from build123d import *

# Parameters (mm, degrees)
F1_DEPTH     = 155
F2_R         = 5
F3_T1_DEPTH  = 145
F3_T3_DEPTH  = 28.172866076
F3_T5_DEPTH  = 18.1728662684
F3_T8_ANGLE  = 90
F3_T10_ANGLE = 90
F3_T12_ANGLE = 88.5674563985
F3_T14_ANGLE = 88.5674563985
F4_R         = 2
F5_R         = 1
F6_R         = 1


# Not quite as in the source:
# - a fillet or chamfer that OpenCascade refuses, or shapes differently, is made with other operations: its cross-section is extruded or revolved along the edge and cut away or added


with BuildPart() as f1:
    # F0 (on Top) → F1 (new body)
    with BuildSketch(Plane.XY):
        Polygon((-2.000000095, 0), (0, 0), (0, 30), (18, 30), (18.999999905, 69.9874980486), (17.0006250026, 70.0374980439), (16.0493903369, 32.000000095), (-2.000000095, 32.000000095), align=None)
    extrude(amount=F1_DEPTH)

    # F2
    f2_edges = [f1.edges().sort_by_distance(p)[0] for p in [
        (16.04939, 32, 77.5),
        (18.000312, 70.012498, 155),
        (18.000312, 70.012498, 0),
    ]]
    fillet(f2_edges, radius=F2_R)

    # F3: fillet of radius 2 on 6 edges, made by hand

    # F3_s2 → F3_t1 (cut)
    with BuildSketch(Plane.XY.offset(5)):
        with BuildLine():
            ThreePointArc((18.999999905, 69.9874980486), (17.5715836938, 69.4372500336), (16.9506250073, 68.0381231415))
            Line((16.9506250073, 68.0381231415), (17.0006250026, 70.0374980439))
            Line((17.0006250026, 70.0374980439), (18.999999905, 69.9874980486))
        make_face()
    extrude(amount=F3_T1_DEPTH, mode=Mode.SUBTRACT)

    # F3_s4 → F3_t3 (cut)
    with BuildSketch(Plane(origin=(1.6360154319, 65.4201701064, 0), x_dir=(0, 0, 1), z_dir=(-0.0249999976, -0.9996874512, 0))):
        with BuildLine():
            ThreePointArc((0, -17.2443741931), (0.5857864376, -15.8301606308), (2, -15.2443741931))
            Line((2, -15.2443741931), (0, -15.2443741931))
            Line((0, -15.2443741931), (0, -17.2443741931))
        make_face()
        with BuildLine():
            ThreePointArc((155, -17.2443741931), (154.4142135624, -15.8301606308), (153, -15.2443741931))
            Line((153, -15.2443741931), (155, -15.2443741931))
            Line((155, -15.2443741931), (155, -17.2443741931))
        make_face()
    extrude(amount=F3_T3_DEPTH, mode=Mode.SUBTRACT)

    # F3_s6 → F3_t5 (cut)
    with BuildSketch(Plane.YZ.offset(-7.000000095)):
        with BuildLine():
            ThreePointArc((30.000000095, 155), (31.4142136574, 154.4142135624), (32.000000095, 153))
            Line((32.000000095, 153), (32.000000095, 155))
            Line((32.000000095, 155), (30.000000095, 155))
        make_face()
        with BuildLine():
            ThreePointArc((30.000000095, 0), (31.4142136574, 0.5857864376), (32.000000095, 2))
            Line((32.000000095, 2), (32.000000095, 0))
            Line((32.000000095, 0), (30.000000095, 0))
        make_face()
    extrude(amount=F3_T5_DEPTH, mode=Mode.SUBTRACT)

    # F3_s7 → F3_t8 (revolve, cut)
    with BuildSketch(Plane.XY.offset(5)):
        with BuildLine():
            ThreePointArc((18.999999905, 69.9874980486), (17.5715836938, 69.4372500336), (16.9506250073, 68.0381231415))
            Line((16.9506250073, 68.0381231415), (17.0006250026, 70.0374980439))
            Line((17.0006250026, 70.0374980439), (18.999999905, 69.9874980486))
        make_face()
    revolve(axis=Axis((16.8756250144, 65.0390607878, 5), (-0.9996874512, 0.0249999976, 0)), revolution_arc=F3_T8_ANGLE, mode=Mode.SUBTRACT)

    # F3_s9 → F3_t10 (revolve, cut)
    with BuildSketch(Plane.XY.offset(150)):
        with BuildLine():
            ThreePointArc((18.999999905, 69.9874980486), (17.5715836938, 69.4372500336), (16.9506250073, 68.0381231415))
            Line((16.9506250073, 68.0381231415), (17.0006250026, 70.0374980439))
            Line((17.0006250026, 70.0374980439), (18.999999905, 69.9874980486))
        make_face()
    revolve(axis=Axis((16.8756250144, 65.0390607878, 150), (0.9996874512, -0.0249999976, 0)), revolution_arc=F3_T10_ANGLE, mode=Mode.SUBTRACT)

    # F3_s11 → F3_t12 (revolve, cut)
    with BuildSketch(Plane(origin=(0.9316938469, 37.2561094255, 0), x_dir=(0, 0, 1), z_dir=(0.0249999976, 0.9996874512, 0))):
        with BuildLine():
            ThreePointArc((155, 17.2443741931), (154.4142135624, 15.8301606308), (153, 15.2443741931))
            Line((153, 15.2443741931), (155, 15.2443741931))
            Line((155, 15.2443741931), (155, 17.2443741931))
        make_face()
    revolve(axis=Axis((11.1728661734, 37.000000095, 155), (0, 0, -1)), revolution_arc=F3_T12_ANGLE, mode=Mode.SUBTRACT)

    # F3_s13 → F3_t14 (revolve, cut)
    with BuildSketch(Plane(origin=(0.9316938469, 37.2561094255, 0), x_dir=(0, 0, 1), z_dir=(0.0249999976, 0.9996874512, 0))):
        with BuildLine():
            ThreePointArc((0, 17.2443741931), (0.5857864376, 15.8301606308), (2, 15.2443741931))
            Line((2, 15.2443741931), (0, 15.2443741931))
            Line((0, 15.2443741931), (0, 17.2443741931))
        make_face()
    revolve(axis=Axis((11.1728661734, 37.000000095, 0), (0, 0, -1)), revolution_arc=F3_T14_ANGLE, mode=Mode.SUBTRACT)

    # F4
    f4_edges = [f1.edges().sort_by_distance(p)[0] for p in [
        (18, 30, 77.5),
    ]]
    fillet(f4_edges, radius=F4_R)

    # F5
    f5_edges = [f1.edges().sort_by_distance(p)[0] for p in [
        (-2, 0, 77.5),
    ]]
    fillet(f5_edges, radius=F5_R)

    # F6
    f6_edges = [f1.edges().sort_by_distance(p)[0] for p in [
        (-2, 32, 77.5),
        (-0.5, 0, 0),
        (-1.707107, 0.292893, 0),
        (-2, 15.5, 0),
        (-0.5, 0, 155),
        (-1.707107, 0.292893, 155),
        (-2, 31.414214, 0.585786),
        (-2, 15.5, 155),
        (-2, 31.414214, 154.414214),
    ]]
    fillet(f6_edges, radius=F6_R)


solid = f1.part
Can you work these out from the model? Positions are in its coordinate system, mm. A direction names the side the tool comes from. Give positions to 0.01 mm unless a question says otherwise; leave off trailing zeros. Loops run counter-clockwise (first coordinate to the right, second up) from the corner with the lowest first, then second, coordinate; pieces in that order, holes last. Notation, with made-up numbers: (22.5, -8.5) -> (29.5, -8.5) arc R28 ccw to (29.5, 10.5) -> close; hole circle Ø9 at (2.25, 60). An arc over 180 degrees is marked (long way). Use one line per item in the form item = value.
1) If we section it at B-B (y = 10.5): Please give me the cut outline in (x, z).
Answers:
outline = (-2, 1) arc R1 ccw to (-1, 0) -> (0, 0) -> (0, 155) -> (-1, 155) arc R1 ccw to (-2, 154) -> close
2) If we section it at C-C (x = 3.5): Please give me the cut outline in (y, z).
Answers:
outline = (30, 0) arc R2 ccw to (32, 2) -> (32, 153) arc R2 ccw to (30, 155) -> close
3) I need wall thicknesses on line 1 along Y through (x, z) = (2.75, 10); line 2 along X through (y, z) = (20, 134.5); line 3 along X through (y, z) = (65.5, 52.5). Which ranges of each line are inside material? Lowest first, please.
Answers:
line_1 = 30 to 32
line_2 = -2 to 0
line_3 = 16.89 to 18.89
4) Will these pins go through, and if not, where does the flat tip stop? pin 1 (8 mm diameter, centred on y = 56.5, z = 21.5, fed in from +X); pin 2 (12 mm diameter, centred on y = 61.5, z = 33.5, fed in from -X); pin 3 (2 mm diameter, centred on x = 3.5, z = 52.5, fed in from +Y); pin 4 (1.5 mm diameter, centred on x = 12.5, y = 29, fed in from +Z).
Answers:
pin_1 = 18.76
pin_2 = 16.64
pin_3 = 32
pin_4 = through
5) For faces 1 (the face through (17.1, 51.1, 0.6)), 2 (the face through (5, 32, 76)), 3 (the face through (0, 15, 76)), 4 (the face through (17.1, 51.1, 154.4)), which set-ups out of +Z, -Z, +X, -X, +Y, -Y let a thin tool reach every point of the face, with its end or its side?
Answers:
face_1 = -Z, -X, +Y
face_2 = +Z, -Z, -X, +Y
face_3 = +Z, -Z, +X, -Y
face_4 = +Z, -X, +Y
